Read the model definition and answer for the solid it produces. Units are mm, in the model's axes. Face numbers are marked on the shaded views. Give positions to 0.01 mm unless a question says otherwise; leave off trailing zeros. Order: outer loops, then holes, each group sorted by start corner. A loop starts at its lowest first (then second) coordinate and runs counter-clockwise, first axis right, second up.
Item 1: A cutting plane is placed at A-A (z = 0). Write down the section's boundary in (x, y).
Item 2: The mould has two halves that part along X. Classify the marked faces 1, 2 and 3: +X half, -X half, draft (parallel to the pull), parting line (faces both ways), or undercut.
Item 3: Find the intervals of material crossed by line 1 along X through (y, z) = (1.8, 35); line 2 along X through (y, z) = (13, 0); line 3 along X through (y, z) = (-1.95, 35), in increasing order.
Item 4: A cutting plane is placed at B-B (x = 74.5). Write down the section's boundary in (y, z), plus the area to 3 significant figures.
Item 5: A cutting plane is placed at C-C (z = 35). State how many separate pieces and enclosed holes the cut face has, plus the area to 3 significant figures.
Item 6: A cutting plane is placed at D-D (y = 15.5). Write down the section's boundary in (x, z), plus the area to 3 significant figures.
Item 7: Given pin 1 Ø5 at (x, y) = (38, 13) entering from +Z; pin 2 Ø10.5 at (x, z) = (-63, 33) entering from +Y; pin 3 Ø1.5 at (y, z) = (13.5, 80) entering from -X, each flat-ended and moving along its own axis, determine where each tip first touches the part or whether it passes through.
from build123d import *

# Parameters (mm, degrees)
SKETCH1_R               = 102.5
BOSS_EXTRUDE2_DEPTH     = 20
SHELL3_T                = 3
SKETCH3_R               = 6.5
BOSS_EXTRUDE8_DEPTH     = 5
SKETCH5_R               = 3
CUT_EXTRUDE2_DEPTH      = 151.534049304
CUT_EXTRUDE2_DEPTH_BACK = 151.534049304


with BuildPart() as part:
    # Sketch1 → Boss-Extrude2 (new body)
    with BuildSketch(Plane(origin=(0, 0, 0), x_dir=(1, 0, 0), z_dir=(0, 1, 0))):
        with Locations(Location((0, 0, 0), (0, 0, 270))):
            Circle(SKETCH1_R)
    extrude(amount=BOSS_EXTRUDE2_DEPTH)

    # Shell3
    shell3_openings = [part.faces().sort_by_distance(p)[0] for p in [
        (0, 20, 0),
    ]]
    offset(amount=SHELL3_T, openings=shell3_openings, kind=Kind.INTERSECTION)

    # Sketch3 → Boss-Extrude8 (add)
    with BuildSketch(Plane(origin=(0, 0, 0), x_dir=(1, 0, 0), z_dir=(0, 1, 0))):
        with BuildLine():
            ThreePointArc((9.5, 70), (0, 79.5), (-9.5, 70))
            Line((-9.5, 70), (-9.5, 5.484827557))
            Line((-9.5, 5.484827557), (-65.371778265, -26.772758664))
            ThreePointArc((-65.371778265, -26.772758664), (-68.849019601, -39.75), (-55.871778265, -43.227241336))
            Line((-55.871778265, -43.227241336), (0, -10.969655115))
            Line((0, -10.969655115), (55.871778265, -43.227241336))
            ThreePointArc((55.871778265, -43.227241336), (68.849019601, -39.75), (65.371778265, -26.772758664))
            Line((65.371778265, -26.772758664), (9.5, 5.484827557))
            Line((9.5, 5.484827557), (9.5, 70))
        make_face()
        with Locations(Location((-60.621778265, -35, 0), (0, 0, 270))):
            Circle(SKETCH3_R, mode=Mode.SUBTRACT)
        with Locations(Location((60.621778265, -35, 0), (0, 0, 270))):
            Circle(SKETCH3_R, mode=Mode.SUBTRACT)
        with Locations(Location((0, 70, 0), (0, 0, 270))):
            Circle(SKETCH3_R, mode=Mode.SUBTRACT)
    extrude(amount=BOSS_EXTRUDE8_DEPTH)

    # Sketch5 → Cut-Extrude2 (cut, two sides)
    with BuildSketch(Plane(origin=(0, 0, 0), x_dir=(1, 0, 0), z_dir=(0, 1, 0))) as cut_extrude2_sk:
        with Locations(Location((0, 70, 0), (0, 0, 270))):
            Circle(SKETCH5_R)
        with Locations(Location((60.621778265, -35, 0), (0, 0, 270))):
            Circle(SKETCH5_R)
        with Locations(Location((-60.621778265, -35, 0), (0, 0, 270))):
            Circle(SKETCH5_R)
    extrude(amount=CUT_EXTRUDE2_DEPTH, mode=Mode.SUBTRACT)
    extrude(cut_extrude2_sk.sketch, amount=-CUT_EXTRUDE2_DEPTH_BACK, mode=Mode.SUBTRACT)


solid = part.part
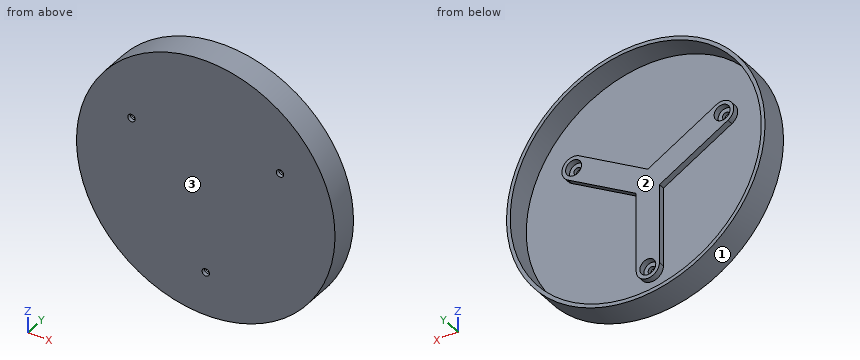
Response values:
1. outline: (-105.5, -3) - (105.5, -3) - (105.5, 20) - (102.5, 20) - (102.5, 0) - (19, 0) - (19, 5) - (-19, 5) - (-19, 0) - (-102.5, 0) - (-102.5, 20) - (-105.5, 20) - close
2. face 1: parting line
2. face 2: undercut
2. face 3: draft
3. line 1: x = -99.53 to -96.34, -70.12 to -67.12, -54.12 to -41.62, 41.62 to 54.12, 67.12 to 70.12, 96.34 to 99.53
3. line 2: x = -105.5 to -102.5, 102.5 to 105.5
3. line 3: x = -99.53 to -63.62, -57.62 to 57.62, 63.62 to 99.53
4. outline: (-3, -74.7) - (20, -74.7) - (20, -70.4) - (0, -70.4) - (0, 70.4) - (20, 70.4) - (20, 74.7) - (-3, 74.7) - close
4. area: 620 mm2
5. separate pieces: 3
5. enclosed holes: 0
5. area: 844 mm2
6. outline: circle Ø211 at (0, 0); hole circle Ø205 at (0, 0)
6. area: 1,960 mm2
7. pin 1: stops at z = 99.35
7. pin 2: stops at y = 5
7. pin 3: stops at x = -69.64
